For this review, take the finished solid that the model builds, in its own axes (mm). Face numbers are marked on the shaded views. A direction names the side the tool comes from. Coordinates: 2 decimals unless noted, no trailing zeros. Order: outer loops, then holes, each group sorted by start corner. A loop starts at its lowest first (then second) coordinate and runs counter-clockwise, first axis right, second up. Notation, with made-up numbers: (85.5, -30.75) -> (109.5, -30.75) arc R23 cw to (109.5, -20.75) -> close; hole circle Ø5 at (14, 89). An arc over 180 degrees is marked (long way). Write item = value, one per line. Start each with the question number.
1) Insertion check: pin 1 Ø4 at (x, y) = (-5, 2) entering from -Z; pin 2 Ø0.5 at (x, y) = (35, -5) entering from +Z; pin 3 Ø5.5 at (x, z) = (-3, 4.5) entering from -Y. Each pin has a flat end and moves straight along its axis. Give the tip position at first contact, or say it passes through.
2) Consider section B-B on z = 5.75. State how many separate pieces and enclosed holes the cut face has, and give its area (3 significant figures).
3) Consider section A-A on x = 12. Give the boundary of the cut face in (y, z).
4) Consider section D-D on y = -8. Give the boundary of the cut face in (x, z), and give its area (3 significant figures).
5) Machinability: for the marked faces 4, 5, 6, 7 and 8, which of the approach directions +Z, -Z, +X, -X, +Y, -Y give a long, thin tool a straight path to every point of the face, cutting with its end or side? Answer none if there is none.
6) Draft analysis for pull direction Y (two halves, no side actions). For the marked faces 1, 2 and 3, state which applies: +Y half, -Y half, draft (parallel to the pull), parting line (faces both ways), or undercut.
7) Wall thickness on probe 1 along Y at (x, z) = (3.1, 4.75); probe 2 along Y at (x, z) = (25.3, 4); probe 3 along X at (y, z) = (-3.75, 4.75): over which ranges is each line inside the solid? List them lowest first. Write a range as [from, to].
8) Consider section C-C on y = -12.5. Give the boundary of the cut face in (x, z), and give its area (3 significant figures).
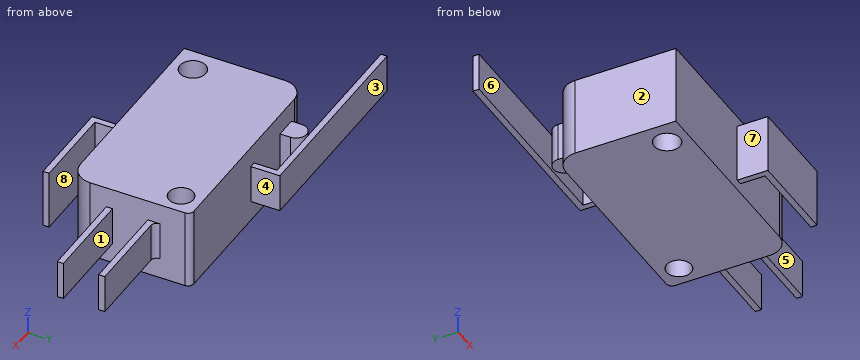
from build123d import *

# Parameters (mm, degrees)
F0_R          = 1.7
F0_R_2        = 1.6
F1_DEPTH      = 10.4
F2_W          = 12.7
F2_H          = 2.7
F2_W_2        = 4
F2_H_2        = 1.35
F3_DEPTH      = 28
F3_DEPTH_BACK = 12.8778
F4_W          = 12
F4_H          = 2.7
F5_DEPTH      = 6.2
F6_T1_DEPTH   = 23.9048285752
F7_R          = 0.762


# Not quite as in the source:
# - a fillet or chamfer that OpenCascade refuses, or shapes differently, is made with other operations: its cross-section is extruded or revolved along the edge and cut away or added
# - a feature names something its author has since deleted; it is built from what else it names


with BuildPart() as f1:
    # F0 (on Top) → F1 (new body)
    with BuildSketch(Plane.XY):
        with BuildLine():
            Line((3.3782, 0), (0, 0))
            Line((0, 0), (0, -15.8))
            Line((0, -15.8), (15, -15.8))
            Line((15, -15.8), (15, -19.8))
            Line((15, -19.8), (27, -19.8))
            Line((27, -19.8), (27, -19))
            Line((27, -19), (15.8, -19))
            Line((15.8, -19), (15.8, -15.8))
            Line((15.8, -15.8), (28, -15.8))
            Line((28, -15.8), (28, -11))
            Line((28, -11), (40, -11))
            Line((40, -11), (40, -10.2))
            Line((40, -10.2), (28, -10.2))
            Line((28, -10.2), (28, -5.6))
            Line((28, -5.6), (40, -5.6))
            Line((40, -5.6), (40, -4.8))
            Line((40, -4.8), (28, -4.8))
            Line((28, -4.8), (28, 0))
            Line((28, 0), (13.31595, 0))
            Line((13.31595, 0), (13.31595, 3.78975))
            Line((13.31595, 3.78975), (-12.8778, 3.78975))
            Line((-12.8778, 3.78975), (-12.8778, 2.996))
            Line((-12.8778, 2.996), (12.5222, 2.996))
            Line((12.5222, 2.996), (12.5222, 0))
            Line((12.5222, 0), (6.1722, 0))
            Line((6.1722, 0), (6.1722, 1.345))
            ThreePointArc((6.1722, 1.345), (4.7752, 2.742), (3.3782, 1.345))
            Line((3.3782, 1.345), (3.3782, 0))
        make_face()
        with Locations((3.1, -13)):
            Circle(F0_R, mode=Mode.SUBTRACT)
        with Locations((25.3, -2.7)):
            Circle(F0_R_2, mode=Mode.SUBTRACT)
    extrude(amount=F1_DEPTH)

    # F2 (on face) → F3 (cut, two sides)
    with BuildSketch(Plane(origin=(0, 0, 0), x_dir=(0, -1, 0), z_dir=(-1, 0, 0))) as f3_sk:
        with Locations((-6.35, 9.05)):
            Rectangle(F2_W, F2_H)
        with Locations((-6.35, 1.35)):
            Rectangle(F2_W, F2_H)
        with Locations((17.8, 9.725)):
            Rectangle(F2_W_2, F2_H_2)
        with Locations((17.8, 0.675)):
            Rectangle(F2_W_2, F2_H_2)
    extrude(amount=-F3_DEPTH, mode=Mode.SUBTRACT)
    extrude(f3_sk.sketch, amount=F3_DEPTH_BACK, mode=Mode.SUBTRACT)

    # F4 (on face) → F5 (cut, through all)
    with BuildSketch(Plane(origin=(0, -4.8, 0), x_dir=(-1, 0, 0), z_dir=(0, 1, 0))):
        with Locations((-34, 9.05)):
            Rectangle(F4_W, F4_H)
        with Locations((-34, 1.35)):
            Rectangle(F4_W, F4_H)
    extrude(amount=-F5_DEPTH, mode=Mode.SUBTRACT)

    # F6: fillet of radius 2.7 on 3 edges, made by hand

    # F6_s2 → F6_t1 (cut)
    with BuildSketch(Plane.XY.offset(-6.7524142876)):
        with BuildLine():
            ThreePointArc((25.2990343146, -15.8004), (27.2091883092, -15.0091883092), (28.0004, -13.0990343146))
            Line((28.0004, -13.0990343146), (28.2705365685, -13.0990343146))
            ThreePointArc((28.2705365685, -13.0990343146), (28.2701365685, -14.4495171573), (28.2701365685, -15.8))
            Line((28.2701365685, -15.8), (28, -16.0701365685))
            ThreePointArc((28, -16.0701365685), (26.6495171573, -16.0701365685), (25.2990343146, -16.0705365685))
            Line((25.2990343146, -16.0705365685), (25.2990343146, -15.8004))
        make_face()
        with BuildLine():
            ThreePointArc((2.7009656854, 0.0004), (0.7908116908, -0.7908116908), (-0.0004, -2.7009656854))
            Line((-0.0004, -2.7009656854), (-0.2705365685, -2.7009656854))
            ThreePointArc((-0.2705365685, -2.7009656854), (-0.2701365685, -1.3504828427), (-0.2701365685, 0))
            Line((-0.2701365685, 0), (0, 0.2701365685))
            ThreePointArc((0, 0.2701365685), (1.3504828427, 0.2701365685), (2.7009656854, 0.2705365685))
            Line((2.7009656854, 0.2705365685), (2.7009656854, 0.0004))
        make_face()
    extrude(amount=F6_T1_DEPTH, mode=Mode.SUBTRACT)

    # F7
    f7_edges = [f1.edges().sort_by_distance(p)[0] for p in [
        (28, 0, 5.2),
        (28, -4.8, 5.2),
    ]]
    fillet(f7_edges, radius=F7_R)


solid = f1.part
Answer sheet:
q1.pin_1 = 2.7
q1.pin_2 = 7.7
q1.pin_3 = 3
q2.separate_pieces = 1
q2.enclosed_holes = 2
q2.area = 484 mm2
q3.outline = (-15.8, 0) -> (0, 0) -> (0, 10.4) -> (-15.8, 10.4) -> close; (3, 2.7) -> (3.79, 2.7) -> (3.79, 7.7) -> (3, 7.7) -> close
q4.outline = (0, 0) -> (28, 0) -> (28, 10.4) -> (0, 10.4) -> close
q4.area = 291 mm2
q5.face_4 = +Z, -Z, +X, +Y
q5.face_5 = +Z, -Z, +X, -Y
q5.face_6 = +Z, -Z, -X
q5.face_7 = +Z, -Z, -X, -Y
q5.face_8 = +Z, -Z, +X
q6.face_1 = undercut
q6.face_2 = draft
q6.face_3 = +Y half
q7.probe_1 = [-15.8, -14.7], [-11.3, 0], [3, 3.79]
q7.probe_2 = [-19.8, -19], [-15.8, -4.3], [-1.1, 0]
q7.probe_3 = [0, 24.09], [26.51, 28]
q8.outline = (0, 0) -> (1.48, 0) -> (1.48, 10.4) -> (0, 10.4) -> close; (4.72, 0) -> (28, 0) -> (28, 10.4) -> (4.72, 10.4) -> close
q8.area = 257 mm2
